```python
from build123d import *

# Parameters (mm, degrees)
F0_R     = 10
F0_R_2   = 0.9
F1_DEPTH = 2


with BuildPart() as f1:
    # F0 (on Top) → F1 (new body)
    with BuildSketch(Plane.XY):
        Circle(F0_R)
        with BuildLine():
            ThreePointArc((-2.517282, -3.108584), (-1.530734, -3.695518), (-0.418114, -3.978088))
            Line((-0.418114, -3.978088), (-0.940756, -8.950697))
            ThreePointArc((-0.940756, -8.950697), (-3.444151, -8.314916), (-5.663884, -6.994314))
            Line((-5.663884, -6.994314), (-2.517282, -3.108584))
        make_face(mode=Mode.SUBTRACT)
        with BuildLine():
            ThreePointArc((-6.994314, -5.663884), (-8.314916, -3.444151), (-8.950697, -0.940756))
            Line((-8.950697, -0.940756), (-3.978088, -0.418114))
            ThreePointArc((-3.978088, -0.418114), (-3.695518, -1.530734), (-3.108584, -2.517282))
            Line((-3.108584, -2.517282), (-6.994314, -5.663884))
        make_face(mode=Mode.SUBTRACT)
        with BuildLine():
            ThreePointArc((0.418114, -3.978088), (1.530734, -3.695518), (2.517282, -3.108584))
            Line((2.517282, -3.108584), (5.663884, -6.994314))
            ThreePointArc((5.663884, -6.994314), (3.444151, -8.314916), (0.940756, -8.950697))
            Line((0.940756, -8.950697), (0.418114, -3.978088))
        make_face(mode=Mode.SUBTRACT)
        with BuildLine():
            Line((6.994314, -5.663884), (3.108584, -2.517282))
            ThreePointArc((3.108584, -2.517282), (3.695518, -1.530734), (3.978088, -0.418114))
            Line((3.978088, -0.418114), (8.950697, -0.940756))
            ThreePointArc((8.950697, -0.940756), (8.314916, -3.444151), (6.994314, -5.663884))
        make_face(mode=Mode.SUBTRACT)
        with BuildLine():
            Line((-6.994314, 5.663884), (-3.108584, 2.517282))
            ThreePointArc((-3.108584, 2.517282), (-3.695518, 1.530734), (-3.978088, 0.418114))
            Line((-3.978088, 0.418114), (-8.950697, 0.940756))
            ThreePointArc((-8.950697, 0.940756), (-8.314916, 3.444151), (-6.994314, 5.663884))
        make_face(mode=Mode.SUBTRACT)
        with BuildLine():
            Line((-0.940756, 8.950697), (-0.418114, 3.978088))
            ThreePointArc((-0.418114, 3.978088), (-1.530734, 3.695518), (-2.517282, 3.108584))
            Line((-2.517282, 3.108584), (-5.663884, 6.994314))
            ThreePointArc((-5.663884, 6.994314), (-3.444151, 8.314916), (-0.940756, 8.950697))
        make_face(mode=Mode.SUBTRACT)
        Circle(F0_R_2, mode=Mode.SUBTRACT)
        with BuildLine():
            ThreePointArc((3.978088, 0.418114), (3.695518, 1.530734), (3.108584, 2.517282))
            Line((3.108584, 2.517282), (6.994314, 5.663884))
            ThreePointArc((6.994314, 5.663884), (8.314916, 3.444151), (8.950697, 0.940756))
            Line((8.950697, 0.940756), (3.978088, 0.418114))
        make_face(mode=Mode.SUBTRACT)
        with BuildLine():
            Line((5.663884, 6.994314), (2.517282, 3.108584))
            ThreePointArc((2.517282, 3.108584), (1.530734, 3.695518), (0.418114, 3.978088))
            Line((0.418114, 3.978088), (0.940756, 8.950697))
            ThreePointArc((0.940756, 8.950697), (3.444151, 8.314916), (5.663884, 6.994314))
        make_face(mode=Mode.SUBTRACT)
    extrude(amount=F1_DEPTH)


solid = f1.part
```
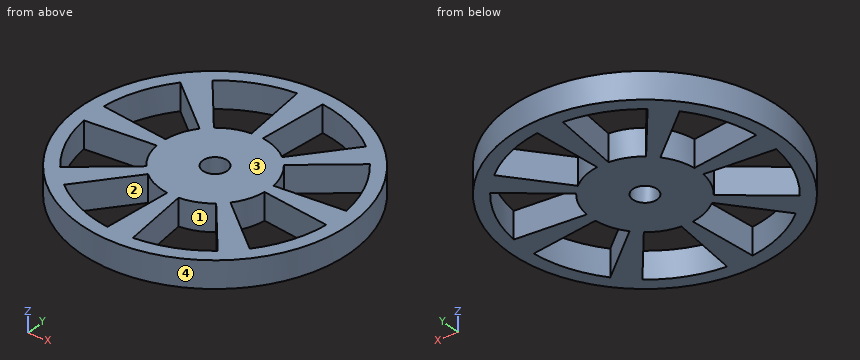
Work out the finished part from the listing and answer in its coordinate system (mm). Face numbers are marked on the shaded views. Round coordinates to 2 decimals unless told otherwise and drop trailing zeros. Loops run counter-clockwise (first coordinate to the right, second up) from the corner with the lowest first, then second, coordinate; pieces in that order, holes last. Notation, with made-up numbers: M 12.25,7 L 16.25,7 A22 ccw 16.25,13 Z; hole C -14.5,29.5 d9. An arc over 180 degrees is marked long. One line per question, with ' | ' between items.
Q1. Find section D-D, the plane x = 3.75. Give the vertices of the cut face in (y, z), then the cut area to 3 significant figures.
Conclusion:
outline: M -9.27,0 L -8.18,0 L -8.18,2 L -9.27,2 Z; M -4.63,0 L -3.04,0 L -3.04,2 L -4.63,2 Z; M -1.39,0 L 1.39,0 L 1.39,2 L -1.39,2 Z; M 3.04,0 L 4.63,0 L 4.63,2 L 3.04,2 Z; M 8.18,0 L 9.27,0 L 9.27,2 L 8.18,2 Z | area: 16.3 mm2
Q2. Find section A-A, the plane y = 0. Give the vertices of the cut face in (x, z).
Conclusion:
outline: M -10,0 L -0.9,0 L -0.9,2 L -10,2 Z; M 0.9,0 L 10,0 L 10,2 L 0.9,2 Z
Q3. This flat-tipped pin is pushed along its axis until it touches: pin 1 Ø2.5 at (x, y) = (0, 0) entering from -Z. Where does it stop, or does it pass through?
Conclusion:
pin 1: stops at z = 0
Q4. Consider line 1 along Y through (x, z) = (0, 1.35); line 2 along X through (y, z) = (2.5, 0.95); line 3 along X through (y, z) = (-2.75, 1.7). Determine where each line is inside the solid, lowest interval first. Write a range as from..to.
Conclusion:
line 1: y = -10..-0.9, 0.9..10 | line 2: x = -9.68..-8.65, -3.12..3.12, 8.65..9.68 | line 3: x = -9.61..-8.57, -3.4..3.4, 8.57..9.61
Q5. Find section C-C, the plane z = 1.3. State how many separate pieces and enclosed holes the cut face has, then the cut area to 3 significant figures.
Conclusion:
separate pieces: 1 | enclosed holes: 9 | area: 162 mm2
Q6. The mould has two halves that part along Y. Classify the marked faces 1, 2, 3 and 4: +Y half, -Y half, draft (parallel to the pull), parting line (faces both ways), or undercut.
Conclusion:
face 1: undercut | face 2: undercut | face 3: draft | face 4: parting line
